Autodesk Inventor part; units mm, degrees
ref_plane "YZ Plane" through (0, 0, 0) normal (1, 0, 0) x (0, 1, 0)
ref_plane "XZ Plane" through (0, 0, 0) normal (0, 1, 0) x (-1, 0, 0)
ref_plane "XY Plane" through (0, 0, 0) normal (0, 0, 1) x (1, 0, 0)
sketch "Sketch1" plane through (0, 0, 0) normal (0, 0, 1) x (1, 0, 0)
  line L0 (120, -15) -> (120, -15)
  line L1 (105, -30) -> (15, -30)
  line L2 (0, -15) -> (0, -15)
  line L3 (13.5, -10) -> (16.5, -10)
  line L4 (16.5, -10) -> (16.5, -20)
  line L5 (16.5, -20) -> (13.5, -20)
  line L6 (13.5, -20) -> (13.5, -10)
  line L7 (103.5, -10) -> (106.5, -10)
  line L8 (106.5, -10) -> (106.5, -20)
  line L9 (106.5, -20) -> (103.5, -20)
  line L10 (103.5, -20) -> (103.5, -10)
  arc A0 (15, 0) -> (0, -15) centre (15, -15) ccw
  arc A1 (0, -15) -> (15, -30) centre (15, -15) ccw
  arc A2 (105, -30) -> (120, -15) centre (105, -15) ccw
  arc A3 (120, -15) -> (105, 0) centre (105, -15) ccw
  line L11 (65, 0) -> (65, -3)
  line L12 (65, -3) -> (55, -3)
  line L13 (55, -3) -> (55, 0)
  line L14 (15, 0) -> (55, 0)
  line L15 (65, 0) -> (105, 0)
  line L16 (90, -13) -> (90, -21)
  line L17 (30, -21) -> (30, -13)
  arc A4 (35, -8) -> (30, -13) centre (35, -13) ccw
  arc A5 (90, -13) -> (85, -8) centre (85, -13) ccw
  arc A6 (85, -26) -> (90, -21) centre (85, -21) ccw
  arc A7 (30, -21) -> (35, -26) centre (35, -21) ccw
  line L18 (62.5, -13) -> (62.5, -21)
  line L19 (57.5, -21) -> (57.5, -13)
  line L20 (35, -8) -> (52.5, -8)
  line L21 (67.5, -8) -> (85, -8)
  line L22 (85, -26) -> (67.5, -26)
  line L23 (52.5, -26) -> (35, -26)
  arc A8 (57.5, -13) -> (52.5, -8) centre (52.5, -13) ccw
  arc A9 (52.5, -26) -> (57.5, -21) centre (52.5, -21) ccw
  arc A10 (62.5, -21) -> (67.5, -26) centre (67.5, -21) ccw
  arc A11 (67.5, -8) -> (62.5, -13) centre (67.5, -13) ccw
  circle A12 centre (6.868, -6.868) radius 1
  circle A13 centre (6.868, -23.132) radius 1
  circle A14 centre (23.132, -23.132) radius 1
  circle A15 centre (23.132, -6.868) radius 1
  circle A16 centre (113.132, -6.868) radius 1
  circle A17 centre (96.868, -6.868) radius 1
  circle A18 centre (96.868, -23.132) radius 1
  circle A19 centre (113.132, -23.132) radius 1
  point P0 (0, 0)
  point P1 (120, 0)
  point P2 (0, -30)
  dimension "d0" = 30
  dimension "d1" = 120
  dimension "d2" = 10
  dimension "d3" = 3
  dimension "d4" = 13.5
  dimension "d5" = 10
  dimension "d6" = 87
  dimension "d7" = 3
  dimension "d8" = 10
  dimension "d9" = 10
  dimension "d10" = 15
  dimension "d11" = 10
  dimension "d12" = 55
  dimension "d13" = 3
  dimension "d18" = 30
  dimension "d19" = 30
  dimension "d20" = 5
  dimension "d23" = 27.5
  dimension "d24" = 27.5
  dimension "d25" = 5
  dimension "d26" = 5
  dimension "d27" = 8
  dimension "d30" = 2
  dimension "d31" = 8.132
  dimension "d32" = 8.132
  dimension "d35" = 360
  dimension "d37" = 2
  dimension "d40" = 8.132
  dimension "d41" = 8.132
  dimension "d44" = 360
  dimension "d48" = 18
  dimension "d50" = 3
  dimension "d51" = 15
extrude "Extrusion4" add sketch "Sketch1" along normal blind 3
properties part number "OpenROV 2_1 Mid Bulkhead"
Geometry: final body of the model. Coordinates: model frame, mm. A direction names the side the tool comes from. Give positions to 0.01 mm unless a question says otherwise; leave off trailing zeros. Loops run counter-clockwise (first coordinate to the right, second up) from the corner with the lowest first, then second, coordinate; pieces in that order, holes last. Notation, with made-up numbers: M -1,-19 L 22,-19 A33 ccw 22,17 Z; hole C -29,69 d3. An arc over 180 degrees is marked long. Put each result on its own line as item: value. Start each with the question number.
1) Cut plane B-B (x = 63.5). Output: boundary loops of the cut face in (y, z), then the cut area to 3 significant figures.
2) Access query for faces 1 (the flat face through (55, -2, 1)), 2 (the flat face through (15, -10, 1)), 3 (the flat face through (59, -15, 0)). Directions: +Z, -Z, +X, -X, +Y, -Y. A direction counts if a zero-diameter tool reaches every point of the face in a straight line with its end or side. Return the directions, or none.
3) Cut plane D-D (x = 10). Output: boundary loops of the cut face in (y, z), then the cut area to 3 significant figures.
4) Pull-direction query (X, two-part tool) for faces 4 (the flat face through (44, -8, 1)), 5 (the flat face through (35, 0, 1)), 6 (the cylindrical face through (120, -15, 1)); classes: pulls with the +X half, pulls with the -X half, needs draft (parallel to the pull), parting line crosses it, or undercut.
5) Cut plane A-A (y = -15). Output: boundary loops of the cut face in (x, z), then the cut area to 3 significant figures.
6) Ray query, line 1 along Y through (x, z) = (68, 2.45); line 2 along X through (y, z) = (-8.5, 1.7); line 3 along Y through (x, z) = (97, 2.85). Return the intervals inside material, ascending.
7) Cut plane C-C (z = 1.45). Give the number of separate pieces and of enclosed holes in the cut face, then the cut area to 3 significant figures.
8) Contact query for flat-ended pins moving along their axis: pin 1 (0.9 mm diameter, centred on y = -13, z = 1.5, fed in from -X); pin 2 (1.5 mm diameter, centred on y = -16, z = 1.5, fed in from +X); pin 3 (1.5 mm diameter, centred on y = -17, z = 1.5, fed in from +X). Output: stop coordinate, or through.
Verdict:
1. outline: M -30,0 L -24,0 L -24,3 L -30,3 Z; M -10,0 L -3,0 L -3,3 L -10,3 Z
1. area: 39.0 mm2
2. face 1: +Z, -Z, +Y
2. face 2: +Z, -Z
2. face 3: -Z, +X, -X, +Y, -Y
3. outline: M -29.14,0 L -0.86,0 L -0.86,3 L -29.14,3 Z
3. area: 84.9 mm2
4. face 4: undercut
4. face 5: needs draft
4. face 6: pulls with the +X half
5. outline: M 0,0 L 13.5,0 L 13.5,3 L 0,3 Z; M 16.5,0 L 30,0 L 30,3 L 16.5,3 Z; M 57.5,0 L 62.5,0 L 62.5,3 L 57.5,3 Z; M 90,0 L 103.5,0 L 103.5,3 L 90,3 Z; M 106.5,0 L 120,0 L 120,3 L 106.5,3 Z
5. area: 177 mm2
6. line 1: -30 to -26, -8 to 0
6. line 2: 1.48 to 32.82, 54.68 to 65.32, 87.18 to 118.52
6. line 3: -30 to -24.12, -22.14 to -7.86, -5.88 to 0
7. separate pieces: 1
7. enclosed holes: 12
7. area: 2,340 mm2
8. pin 1: x = 0.08
8. pin 2: x = 120
8. pin 3: x = 119.95
